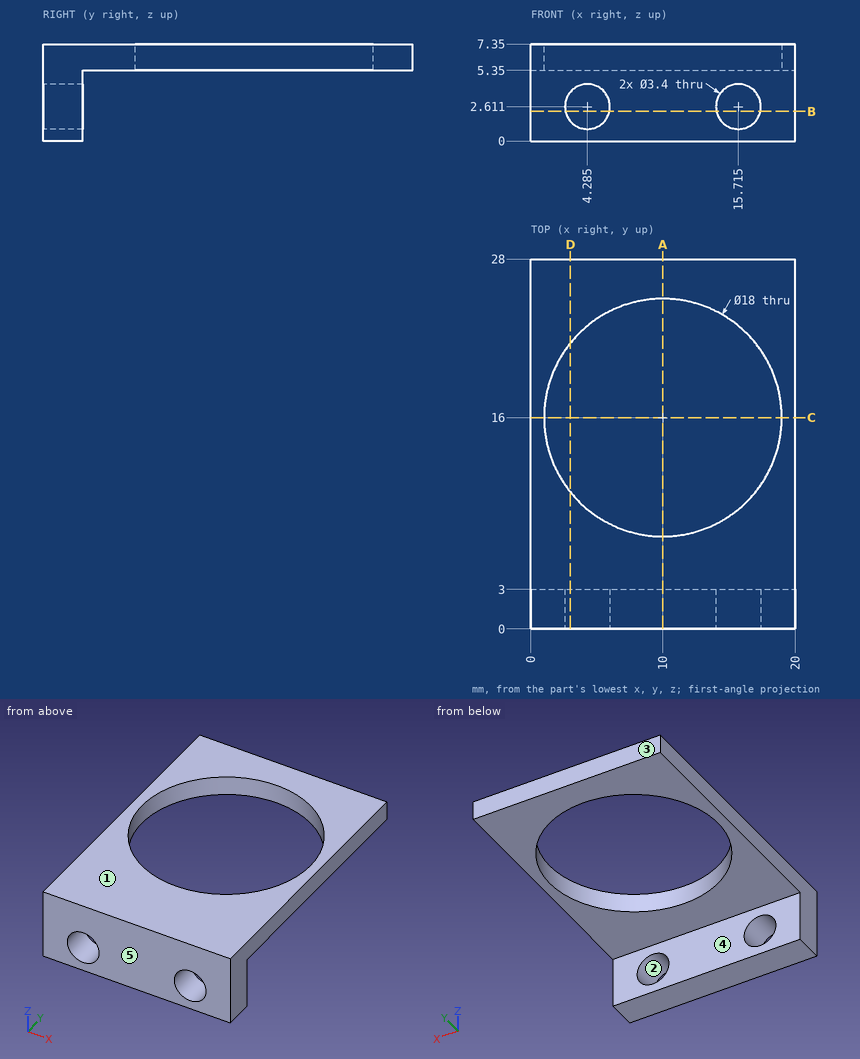
Source: three-view drawing plus pictorial views. Frame: mm from the lowest corner of the part. A direction names the side the tool comes from. Give positions to 0.01 mm unless a question says otherwise; leave off trailing zeros. Order: outer loops, then holes, each group sorted by start corner. A loop starts at its lowest first (then second) coordinate and runs counter-clockwise, first axis right, second up.
1. Section B-B on z = 2.25. Return the cut outline in (x, y).
Derived:
outline: (0, 0) - (2.62, 0) - (2.62, 3) - (0, 3) - close; (5.95, 0) - (14.05, 0) - (14.05, 3) - (5.95, 3) - close; (17.38, 0) - (20, 0) - (20, 3) - (17.38, 3) - close
2. Section D-D on x = 3. Return the cut outline in (y, z).
Derived:
outline: (0, 0) - (3, 0) - (3, 1.5) - (0, 1.5) - close; (0, 3.72) - (3, 3.72) - (3, 5.35) - (10.34, 5.35) - (10.34, 7.35) - (0, 7.35) - close; (21.66, 5.35) - (28, 5.35) - (28, 7.35) - (21.66, 7.35) - close
3. Reachability of the marked faces 4 and 5 from +Z, -Z, +X, -X, +Y, -Y: full face, straight path, thin tool, end or side. Return the list, or none.
Derived:
face 4: -Z, +X, -X, +Y
face 5: +Z, -Z, +X, -X, -Y
4. Section C-C on y = 16. Return the cut outline in (x, z).
Derived:
outline: (0, 5.35) - (1, 5.35) - (1, 7.35) - (0, 7.35) - close; (19, 5.35) - (20, 5.35) - (20, 7.35) - (19, 7.35) - close
5. Pin query (flat end, axial travel): pin 1 (8 mm diameter, centred on x = 11.5, y = 15.5, fed in from -Z); pin 2 (1.6 mm diameter, centred on x = 12, z = 3.5, fed in from +Y). Return the tip coordinate at first contact, or that it passes through.
Derived:
pin 1: passes through
pin 2: stops at y = 3
6. Section A-A on x = 10. Return the cut outline in (y, z).
Derived:
outline: (0, 0) - (3, 0) - (3, 5.35) - (7, 5.35) - (7, 7.35) - (0, 7.35) - close; (25, 5.35) - (28, 5.35) - (28, 7.35) - (25, 7.35) - close
7. Material intervals for L1, parallel to Y at x = 9, z = 2; L2, parallel to Z at x = 14.75, y = 2.25; L3, parallel to X at y = 12, z = 5.5, sorted ascending.
Derived:
L1: y = 0 to 3
L2: z = 0 to 1.21, 4.01 to 7.35
L3: x = 0 to 1.94, 18.06 to 20
8. Mould query, pull axis Z, two halves, no side actions, for the marked faces 1, 2 and 3. Classes: released by +Z, released by -Z, zero draft, split by the parting line, or undercut.
Derived:
face 1: released by +Z
face 2: undercut
face 3: zero draft
